Job drawing, mm, ordinate dimensions from the low corner. One solid piece. A direction names the side the tool comes from. Round coordinates to 2 decimals unless told otherwise and drop trailing zeros. Order: outer loops, then holes, each group sorted by start corner. A loop starts at its lowest first (then second) coordinate and runs counter-clockwise, first axis right, second up. Notation, with made-up numbers: (-7, -8.5) -> (0, -8.5) arc R23 ccw to (0, 13.5) -> close; hole circle Ø8 at (4.25, -29.75). An arc over 180 degrees is marked (long way). Return JSON: item names as keys, results as strings. Group by question number.
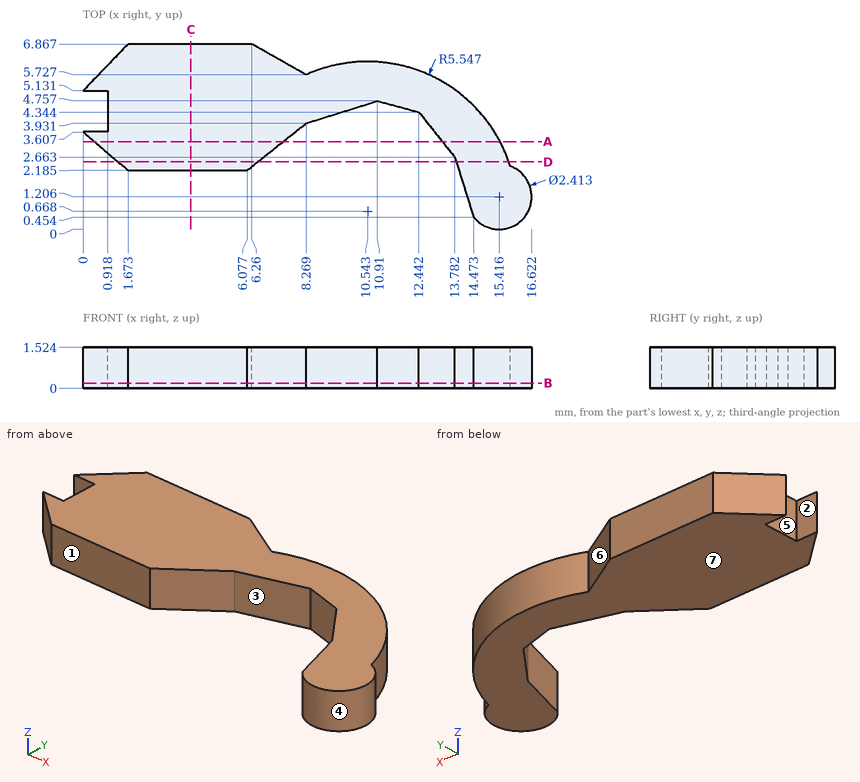
(1) Saw through at D-D, the plane y = 2.5. List the corners of the cut face in (x, z).
(2) Probe L1, parallel to X at y = 2.25, z = 1.15 (1 decimal); L2, parallel to Y at x = 6, z = 0.8 (1 decimal); L3, parallel to X at y = 2.5, z = 0.45 (1 decimal). List the from-to ranges inside material, lowest first. Write a range as [from, to].
(3) Saw through at C-C, the plane x = 4. List the corners of the cut face in (y, z) (1 decimal).
(4) Pin check, flat tips, straight feed: P1, Ø0.5, axis at x = 0.5, z = 1, coming from the -Y side; P2, Ø0.8, axis at x = 5, z = 0.5, coming from the -Y side (1 decimal). Stop position of each tip, or through.
(5) Mould opens along X. For the marked faces 4, 5, 6 and 7 say: pulls with the +X half, pulls with the -X half, needs draft (parallel to the pull), parting line crosses it, or undercut.
(6) Tool access for the marked faces 1, 2 and 3: list every direction of +Z, -Z, +X, -X, +Y, -Y with a clear straight run to the whole face (end or side of a thin tool).
(7) Saw through at A-A, the plane y = 3.25. List the corners of the cut face in (x, z).
(8) Saw through at B-B, the plane z = 0.2. List the corners of the cut face in (x, y) (1 decimal).
Results are:
{
 "1": {"outline": "(1.3, 0) -> (6.47, 0) -> (6.47, 1.52) -> (1.3, 1.52) -> close; (13.83, 0) -> (15.78, 0) -> (15.78, 1.52) -> (13.83, 1.52) -> close"},
 "2": {"L1": "x = [1.6, 6.2], [13.9, 16]", "L2": "y = [2.2, 6.9]", "L3": "x = [1.3, 6.5], [13.8, 15.8]"},
 "3": {"outline": "(2.2, 0) -> (6.9, 0) -> (6.9, 1.5) -> (2.2, 1.5) -> close"},
 "4": {"P1": "stops at y = 2.97", "P2": "stops at y = 2.2"},
 "5": {"face 4": "parting line crosses it", "face 5": "pulls with the -X half", "face 6": "undercut", "face 7": "needs draft"},
 "6": {"face 1": "+Z, -Z, -X, -Y", "face 2": "+Z, -Z, -X", "face 3": "+Z, -Z, -Y"},
 "7": {"outline": "(0.42, 0) -> (7.41, 0) -> (7.41, 1.52) -> (0.42, 1.52) -> close; (13.31, 0) -> (15.45, 0) -> (15.45, 1.52) -> (13.31, 1.52) -> close"},
 "8": {"outline": "(0, 3.6) -> (1.7, 2.2) -> (6.1, 2.2) -> (8.3, 3.9) -> (10.9, 4.8) -> (12.4, 4.3) -> (13.8, 2.7) -> (14.5, 0.5) arc R1.2 ccw (long way) to (15.8, 2.3) arc R5.5 ccw to (8.3, 5.7) -> (6.3, 6.9) -> (1.7, 6.9) -> (0, 5.1) -> (0.9, 5.1) -> (0.9, 3.6) -> close"}
}
